Print and shaded views of the part. All mm, measured from the part's lowest x, y and z. Coordinates: 2 decimals unless noted, no trailing zeros. Loops run counter-clockwise (first coordinate to the right, second up) from the corner with the lowest first, then second, coordinate; pieces in that order, holes last.
1) Wall check: line 1 along Z through (x, y) = (106, 5.5) (1 decimal); line 2 along Z through (x, y) = (260, 9.25) (1 decimal); line 3 along X through (y, z) = (9.25, 90) (1 decimal). Give the ranges that are in metal, low to high.
2) Saw through at B-B, the plane y = 7.5. Give the number of separate pieces and of enclosed holes in the cut face, and give its area (3 significant figures).
3) Saw through at C-C, the plane z = 288. Write the cut outline in (x, y), and give its area (3 significant figures).
4) Saw through at A-A, the plane x = 335. Write the cut outline in (y, z).
5) Pin check, flat tips, straight feed: pin 1 Ø4 at (y, z) = (3, 98) entering from -X (1 decimal); pin 2 Ø6 at (x, y) = (246.5, 6) entering from -Z; pin 3 Ø2 at (y, z) = (6, 179.5) entering from +X. Stop position of each tip, or through.
6) Saw through at D-D, the plane x = 57.5. Write the cut outline in (y, z) (1 decimal), and give its area (3 significant figures).
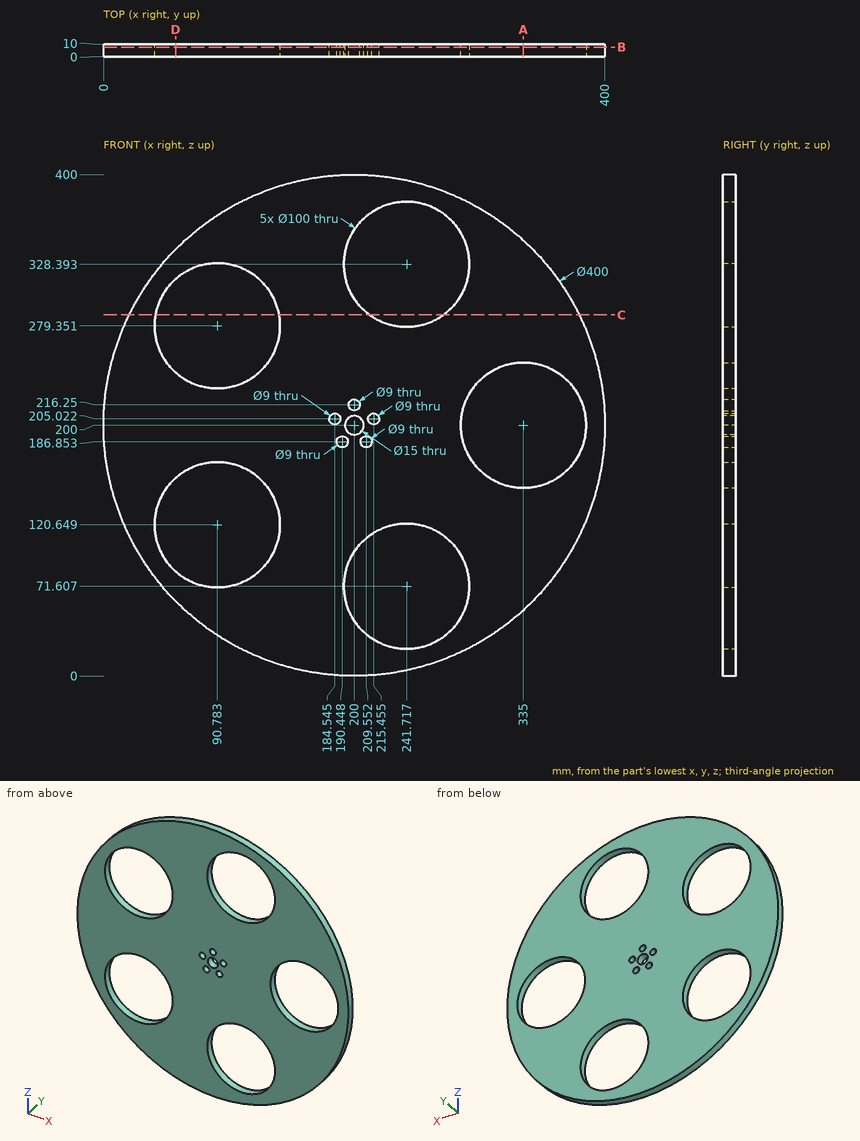
Data:
1. line 1: z = 23.5 to 73, 168.3 to 231.7, 327 to 376.5
1. line 2: z = 9.2 to 25.1, 118.1 to 281.9, 374.9 to 390.8
1. line 3: x = 33 to 51.3, 130.3 to 195.2, 288.2 to 367
2. separate pieces: 1
2. enclosed holes: 11
2. area: 85,900 mm2
3. outline: (20.4, 0) - (41.54, 0) - (41.54, 10) - (20.4, 10) - close; (140.03, 0) - (212.25, 0) - (212.25, 10) - (140.03, 10) - close; (271.19, 0) - (379.6, 0) - (379.6, 10) - (271.19, 10) - close
3. area: 2,020 mm2
4. outline: (0, 52.44) - (10, 52.44) - (10, 150) - (0, 150) - close; (0, 250) - (10, 250) - (10, 347.56) - (0, 347.56) - close
5. pin 1: stops at x = 26.8
5. pin 2: stops at z = 4.79
5. pin 3: stops at x = 399.05
6. outline: (0, 59.7) - (10, 59.7) - (10, 83.3) - (0, 83.3) - close; (0, 158) - (10, 158) - (10, 242) - (0, 242) - close; (0, 316.7) - (10, 316.7) - (10, 340.3) - (0, 340.3) - close
6. area: 1,310 mm2
